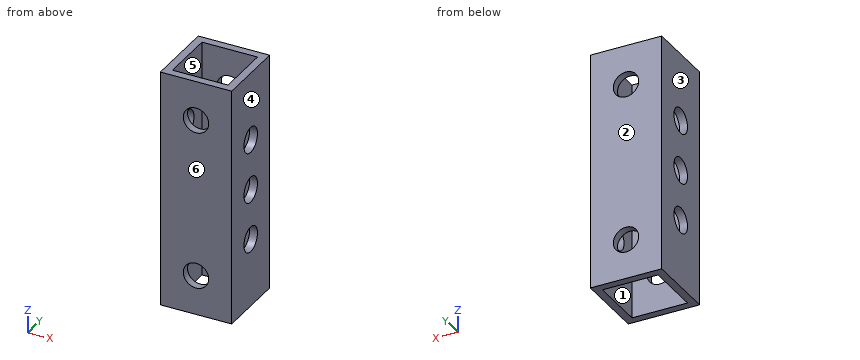
Autodesk Inventor part; units mm, degrees
ref_plane "YZ Plane" through (0, 0, 0) normal (1, 0, 0) x (0, 1, 0)
ref_plane "XZ Plane" through (0, 0, 0) normal (0, 1, 0) x (-1, 0, 0)
ref_plane "XY Plane" through (0, 0, 0) normal (0, 0, 1) x (1, 0, 0)
sketch "スケッチ1" plane through (0, 0, 0) normal (0, 0, 1) x (1, 0, 0)
  line L0 (4.5, -4.5) -> (-4.5, -4.5)
  line L1 (-4.5, -4.5) -> (-4.5, 4.5)
  line L2 (-4.5, 4.5) -> (4.5, 4.5)
  line L3 (4.5, 4.5) -> (4.5, -4.5)
  line L4 (4.5, -4.5) -> (-4.5, 4.5) construction
  line L5 (-4.5, -4.5) -> (4.5, 4.5) construction
  point P0 (0, 0)
  dimension "d0" = 9
  dimension "d1" = 9
extrude "押し出し1" add sketch "スケッチ1" along normal blind 30
shell "シェル1" thickness 1 removed faces 2 at (1.5, -1.5, 0) at (1.5, -1.5, 30)
sketch "スケッチ2" plane through (-4.5, 4.5, 0) normal (0, 1, 0) x (1, 0, 0)
  line L0 (0, 0) -> (9, 0)
  point P0 (4.5, 0)
  point P1 (4.5, -5)
  point P2 (4.5, -25)
  point P3 (4.5, 0)
  dimension "d5" = 20
  dimension "d6" = 5
hole "穴1" at (0, 4.5, 5) at (0, 4.5, 25) direction (0, -1, 0) diameter 3.2 end through all
sketch "スケッチ3" plane through (4.5, -4.5, 0) normal (1, 0, 0) x (0, 0, -1)
  line L0 (0, 9) -> (0, 0)
  line L1 (0, 9) -> (-30, 9)
  line L2 (-30, 0) -> (-30, 9)
  line L3 (0, 0) -> (-30, 0)
  point P0 (0, 4.5)
  point P1 (-15, 4.5)
  point P2 (-15, 9)
  point P3 (0, 4.5)
  point P4 (-8.6, 4.5)
  point P5 (-21.4, 4.5)
  dimension "d21" = 6.4
  dimension "d22" = 6.4
hole "穴2" at (4.5, 0, 15) at (4.5, 0, 8.6) at (4.5, 0, 21.4) direction (-1, 0, 0) diameter 3.2 end through all
properties part number "SqPipeminin"
CAD build for the part. Positions are in the model's coordinates, mm. Face numbers are marked on the shaded views. A direction names the side the tool comes from. Round coordinates to 2 decimals unless told otherwise and drop trailing zeros. Write each loop counter-clockwise with the first axis right and the second up, starting at its lowest first coordinate (ties: lowest second). Pieces come first, ordered by that corner, then holes. Notation, with made-up numbers: M 35,42.5 L 44,42.5 A14 cw 44,68.5 Z; hole C -5,38 d3. An arc over 180 degrees is marked long. Use a Markdown table: item, result. Add a question column.
1. 3-axis set-ups, long thin cutter, end or side, ignore diameter. For the marked faces 5 and 6: which of +Z, -Z, +X, -X, +Y, -Y reach the whole face in a straight line?
2. Pull direction X, two halves, no side cores. Call the marked faces 1, 2, 3 and 4: released by +X, released by -X, zero draft, split by the parting line, or undercut.
3. Slice it at B-B on x = -2. Give the cut face in (y, z), then the cut area to 3 significant figures.
4. Slice it at A-A on y = 0. Give the number of separate pieces and of enclosed holes in the cut face, then the cut area to 3 significant figures.
5. Slice it at C-C on z = 5. Give the cut face in (x, y).
6. Drill centre lines: probe 1 along Z at (x, y) = (4.1, 0); probe 2 along Z at (x, y) = (0, 4.05); probe 3 along X at (y, z) = (3.8, 25). Where is each one in solid material? Low to high.
Reply:
| question | item | result |
|---|---|---|
| 1 | face 5 | +Z, -Z |
| 1 | face 6 | +Z, -Z, +X, -X, -Y |
| 2 | face 1 | undercut |
| 2 | face 2 | zero draft |
| 2 | face 3 | released by -X |
| 2 | face 4 | released by +X |
| 3 | outline | M -4.5,0 L -3.5,0 L -3.5,30 L -4.5,30 Z; M 3.5,0 L 4.5,0 L 4.5,30 L 3.5,30 Z |
| 3 | area | 60.0 mm^2 |
| 4 | separate pieces | 8 |
| 4 | enclosed holes | 0 |
| 4 | area | 40.8 mm^2 |
| 5 | outline | M -4.5,-4.5 L -1.6,-4.5 L -1.6,-3.5 L -3.5,-3.5 L -3.5,3.5 L -1.6,3.5 L -1.6,4.5 L -4.5,4.5 Z; M 1.6,-4.5 L 4.5,-4.5 L 4.5,4.5 L 1.6,4.5 L 1.6,3.5 L 3.5,3.5 L 3.5,-3.5 L 1.6,-3.5 Z |
| 6 | probe 1 | z = 0 to 7, 10.2 to 13.4, 16.6 to 19.8, 23 to 30 |
| 6 | probe 2 | z = 0 to 3.4, 6.6 to 23.4, 26.6 to 30 |
| 6 | probe 3 | x = -4.5 to -1.6, 1.6 to 4.5 |
